The model under review builds one solid part; all positions refer to its coordinate system, in mm. A direction names the side the tool comes from. Round coordinates to 2 decimals unless told otherwise and drop trailing zeros. Order: outer loops, then holes, each group sorted by start corner. A loop starts at its lowest first (then second) coordinate and runs counter-clockwise, first axis right, second up. Notation, with made-up numbers: M -9,-6 L 25,-6 A7 ccw 25,4 Z; hole C -21.5,-37 d7. An arc over 180 degrees is marked long. Answer as a JSON object with one key per item and string values. Group by question number.
1) Consider section A-A, the plane y = 0. Write out the cut boundary in (x, z).
2) Consider section D-D, the plane y = 2. Write out the cut boundary in (x, z), then the cut area to 3 significant figures.
3) Consider section C-C, the plane z = 4.75. Write out the cut boundary in (x, y), then the cut area to 3 significant figures.
4) Insertion check: pin 1 Ø2 at (y, z) = (-1.5, 13.5) entering from +X; pin 2 Ø1.1 at (x, y) = (0, -1) entering from +Z; pin 3 Ø1.5 at (y, z) = (1, 9.5) entering from +X. Each pin has a flat end and moves straight along its axis. Give the tip position at first contact, or say it passes through.
5) To check wall thickness, follow line 1 (Y direction, x = 0, z = 13.5); line 2 (Y direction, x = 0, z = 2.3); line 3 (Z direction, x = 1.7, y = 0.4). State the ranges of each line that lie inside material, in increasing order.
6) For faces 4 (the cylindrical face through (1.717, 0.541, 11.457)), 5 (the flat face through (-1, 2, 20)), list the 3-axis set-ups (+Z, -Z, +X, -X, +Y, -Y) from which the entire face can be reached by the end or side of a thin tool; tool diameter is ignored.
7) The part is to be moulded in two halves that separate along Y. For faces 1 (the flat face through (-1, 1, 3.15)), 2 (the flat face through (-1, -1, 0)), 3 (the cylindrical face through (-0.54, -2.44, 9.86)), say which applies: +Y half, -Y half, draft (parallel to the pull), parting line (faces both ways), or undercut.
```python
from build123d import *

# Parameters (mm, degrees)
CROQUIS1_R                 = 2.5
CROQUIS1_R_2               = 1.8
SALIENTE_EXTRUIR1_DEPTH    = 20
CROQUIS3_R                 = 1.8
SALIENTE_EXTRUIR2_DEPTH    = 3.15
CORTAR_EXTRUIR1_DEPTH      = 21.310096012
CORTAR_EXTRUIR1_DEPTH_BACK = 21.310096012
CROQUIS4_R                 = 1.12


with BuildPart() as part:
    # Croquis1 → Saliente-Extruir1 (new body)
    with BuildSketch(Plane.XY):
        Circle(CROQUIS1_R)
        Circle(CROQUIS1_R_2, mode=Mode.SUBTRACT)
    extrude(amount=SALIENTE_EXTRUIR1_DEPTH)

    # Croquis3 → Saliente-Extruir2 (add)
    with BuildSketch(Plane(origin=(0, 0, 0), x_dir=(-1, 0, 0), z_dir=(0, 0, -1))):
        Circle(CROQUIS3_R)
    extrude(amount=-SALIENTE_EXTRUIR2_DEPTH)

    # Croquis4 → Cortar-Extruir1 (cut, two sides: drawn at the far end of the back side and taken through both)
    with BuildSketch(Plane(origin=(0, 0, 0), x_dir=(-1, 0, 0), z_dir=(0, 0, -1)).offset(-CORTAR_EXTRUIR1_DEPTH_BACK)):
        Circle(CROQUIS4_R)
    extrude(amount=CORTAR_EXTRUIR1_DEPTH + CORTAR_EXTRUIR1_DEPTH_BACK, mode=Mode.SUBTRACT)


solid = part.part
```
Results list:
{
 "1": {"outline": "M -2.5,0 L -1.12,0 L -1.12,3.15 L -1.8,3.15 L -1.8,20 L -2.5,20 Z; M 1.12,0 L 2.5,0 L 2.5,20 L 1.8,20 L 1.8,3.15 L 1.12,3.15 Z"},
 "2": {"outline": "M -1.5,0 L 1.5,0 L 1.5,20 L -1.5,20 Z", "area": "60.0 mm^2"},
 "3": {"outline": "C 0,0 d5; hole C 0,0 d3.6", "area": "9.46 mm^2"},
 "4": {"pin 1": "x = 2.45", "pin 2": "z = 3.15", "pin 3": "x = 2.49"},
 "5": {"line 1": "-2.5 to -1.8, 1.8 to 2.5", "line 2": "-2.5 to -1.12, 1.12 to 2.5", "line 3": "0 to 3.15"},
 "6": {"face 4": "+Z", "face 5": "+Z, +X, -X, +Y, -Y"},
 "7": {"face 1": "undercut", "face 2": "draft", "face 3": "parting line"}
}
